The model under review builds one solid part; all positions refer to its coordinate system, in mm. A direction names the side the tool comes from. Give positions to 0.01 mm unless a question says otherwise; leave off trailing zeros. Order: outer loops, then holes, each group sorted by start corner. A loop starts at its lowest first (then second) coordinate and runs counter-clockwise, first axis right, second up. Notation, with made-up numbers: (-16, 86.25) - (42, 86.25) arc R9 ccw to (42, 93.25) - close; hole circle Ø4 at (83, 24.5). An arc over 180 degrees is marked (long way). Use CSV: the item, a comma, the result in double quotes.
Solid Edge part; units mm, degrees
sketch "Sketch1" plane through (0, 0, 0) normal (0, 1, 0) x (-1, 0, 0)
  line L0 (50, -150) -> (50, 150)
  line L1 (50, 150) -> (-50, 150)
  line L2 (-50, 150) -> (-50, -150)
  line L3 (-50, -150) -> (50, -150)
extrude "Protrusion1" add sketch "Sketch1" against normal blind 100
sketch "Sketch2" plane through (0, 0, 0) normal (0, 1, 0) x (1, 0, 0)
  line L0 (-25, 100) -> (-25, -100)
  line L1 (-25, -100) -> (25, -100)
  line L2 (25, -100) -> (25, 100)
  line L3 (25, 100) -> (-25, 100)
extrude "ExtrudedProtrusion_4" add sketch "Sketch2" along normal blind 1800
sketch "Sketch3" plane through (0, 1800, 0) normal (0, 1, 0) x (1, 0, 0)
  line L0 (50, 150) -> (50, -150)
  line L1 (50, -150) -> (-50, -150)
  line L2 (-50, -150) -> (-50, 150)
  line L3 (-50, 150) -> (50, 150)
extrude "ExtrudedProtrusion_5" add sketch "Sketch3" along normal blind 100
properties material "Aluminum, 1060"
Item 1: Take a section at C-C, the plane z = 68. Give the boundary of the cut face in (x, y).
Results list:
outline,"(-50, -100) - (50, -100) - (50, 0) - (25, 0) - (25, 1800) - (50, 1800) - (50, 1900) - (-50, 1900) - (-50, 1800) - (-25, 1800) - (-25, 0) - (-50, 0) - close"
Item 2: Wall thickness on L1, parallel to Y at x = 41, z = -86; L2, parallel to Z at x = 15, y = 1258.5; L3, parallel to X at y = 481.5, z = 52: over which ranges is each line inside the solid? List them lowest first.
Results list:
L1,"y = -100 to 0, 1800 to 1900"
L2,"z = -100 to 100"
L3,"x = -25 to 25"
Item 3: Take a section at B-B, the plane x = 5.5. Give the boundary of the cut face in (y, z).
Results list:
outline,"(-100, -150) - (0, -150) - (0, -100) - (1800, -100) - (1800, -150) - (1900, -150) - (1900, 150) - (1800, 150) - (1800, 100) - (0, 100) - (0, 150) - (-100, 150) - close"
Item 4: Mouldability with a two-part tool opening along Y and no side actions: class faces 1 (the face through (-25, 887, -1)), 2 (the face through (1, -100, -2)), 3 (the face through (-1, -49, 150)) as pulls with the +Y half, pulls with the -Y half, needs draft (parallel to the pull), parting line crosses it, or undercut.
Results list:
face 1,"undercut"
face 2,"pulls with the -Y half"
face 3,"needs draft"
Item 5: Take a section at D-D, the plane y = 290. Give the boundary of the cut face in (x, z), and give its area (3 significant figures).
Results list:
outline,"(-25, -100) - (25, -100) - (25, 100) - (-25, 100) - close"
area,"10,000 mm2"
Item 6: Tool access review of faces 4 (the face through (25, 887, 1)), 5 (the face through (0, 887, -100)), 6 (the face through (0, 887, 100)): name each direction out of +Z, -Z, +X, -X, +Y, -Y from which nothing blocks a thin tool from reaching the whole face with its end or side.
Results list:
face 4,"+Z, -Z, +X"
face 5,"-Z, +X, -X"
face 6,"+Z, +X, -X"
Item 7: Take a section at A-A, the plane z = -124.5. Give the boundary of the cut face in (x, y).
Results list:
outline,"(-50, -100) - (50, -100) - (50, 0) - (-50, 0) - close; (-50, 1800) - (50, 1800) - (50, 1900) - (-50, 1900) - close"
Item 8: Clearance check with flat-ended pins moving along their axes: pin 1 (2 mm diameter, centred on x = -0.5, y = 398.5, fed in from +Z); pin 2 (8 mm diameter, centred on y = 1522.5, z = -47, fed in from +X); pin 3 (6 mm diameter, centred on y = 1678.5, z = 88.5, fed in from -X). State where each tip first meets the part, or that it passes through.
Results list:
pin 1,"stops at z = 100"
pin 2,"stops at x = 25"
pin 3,"stops at x = -25"
